from build123d import *

# Parameters (mm, degrees)
SKETCH1_W           = 5
SKETCH1_H           = 6.5
SKETCH1_W_2         = 29.5
SKETCH1_H_2         = 9.25
BOSS_EXTRUDE1_DEPTH = 1.62
FILLET1_R           = 10.16
SKETCH1_3_W         = 5
SKETCH1_3_H         = 6.5
BOSS_EXTRUDE2_DEPTH = 7
SKETCH2_R           = 1.5
CUT_EXTRUDE1_DEPTH  = 1.62
SKETCH3_W           = 20
SKETCH3_H           = 7
BOSS_EXTRUDE3_DEPTH = 6


with BuildPart() as part:
    # Sketch1 → Boss-Extrude1 (new body)
    # profile 1 of 7: a face of its own
    with BuildSketch(Plane(origin=(0, 0, 0), x_dir=(1, 0, 0), z_dir=(0, 1, 0))):
        Polygon((-38.5, 4.625), (-14.75, 4.625), (14.75, 4.625), (38.5, 4.625), (38.5, 13.875), (-38.5, 13.875), align=None)
        with Locations((-31.9999868, 9.25)):
            Rectangle(SKETCH1_W, SKETCH1_H, mode=Mode.SUBTRACT)
        with Locations((-15.9999934, 9.25)):
            Rectangle(SKETCH1_W, SKETCH1_H, mode=Mode.SUBTRACT)
        with Locations((0, 9.25)):
            Rectangle(SKETCH1_W, SKETCH1_H, mode=Mode.SUBTRACT)
        with Locations((15.9999934, 9.25)):
            Rectangle(SKETCH1_W, SKETCH1_H, mode=Mode.SUBTRACT)
        with Locations((31.9999868, 9.25)):
            Rectangle(SKETCH1_W, SKETCH1_H, mode=Mode.SUBTRACT)
    # profile 2 of 7: a face of its own
    with BuildSketch(Plane(origin=(0, 0, 0), x_dir=(1, 0, 0), z_dir=(0, 1, 0))):
        with Locations((-31.9999868, 9.25)):
            Rectangle(SKETCH1_W, SKETCH1_H)
    # profile 3 of 7: a face of its own
    with BuildSketch(Plane(origin=(0, 0, 0), x_dir=(1, 0, 0), z_dir=(0, 1, 0))):
        with Locations((-15.9999934, 9.25)):
            Rectangle(SKETCH1_W, SKETCH1_H)
    # profile 4 of 7: a face of its own
    with BuildSketch(Plane(origin=(0, 0, 0), x_dir=(1, 0, 0), z_dir=(0, 1, 0))):
        Rectangle(SKETCH1_W_2, SKETCH1_H_2)
    # profile 5 of 7: a face of its own
    with BuildSketch(Plane(origin=(0, 0, 0), x_dir=(1, 0, 0), z_dir=(0, 1, 0))):
        with Locations((0, 9.25)):
            Rectangle(SKETCH1_W, SKETCH1_H)
    # profile 6 of 7: a face of its own
    with BuildSketch(Plane(origin=(0, 0, 0), x_dir=(1, 0, 0), z_dir=(0, 1, 0))):
        with Locations((15.9999934, 9.25)):
            Rectangle(SKETCH1_W, SKETCH1_H)
    # profile 7 of 7: a face of its own
    with BuildSketch(Plane(origin=(0, 0, 0), x_dir=(1, 0, 0), z_dir=(0, 1, 0))):
        with Locations((31.9999868, 9.25)):
            Rectangle(SKETCH1_W, SKETCH1_H)
    extrude(amount=BOSS_EXTRUDE1_DEPTH)

    # Fillet1
    # the kernel refuses this fillet: 10.16 mm, written as the material it adds along each edge
    with BuildSketch(Plane(origin=(14.75, 0, -4.625), x_dir=(0, 0, 1), z_dir=(0, 1, 0))) as fillet1_piece_1:
        with BuildLine():
            CenterArc((10.16, 10.119164985), FILLET1_R, 180, 84.861306661)
            Line((0, 10.119164985), (-0.2032, 10.119164985))
            Line((-0.2032, 10.119164985), (-0.2032, 0))
            Line((-0.2032, 0), (0, -0.2032))
            ThreePointArc((0, -0.2032), (4.625, -0.2032), (9.2318, -0.2023833))
            Line((9.2318, -0.2023833), (9.25, 0))
        make_face()
    extrude(amount=1.62)
    with BuildSketch(Plane(origin=(-14.75, 0, -4.625), x_dir=(-1, 0, 0), z_dir=(0, 1, 0))) as fillet1_piece_2:
        with BuildLine():
            CenterArc((10.119164985, 10.16), FILLET1_R, 185.138693339, 84.861306661)
            Line((0, 9.25), (-0.2023833, 9.2318))
            ThreePointArc((-0.2023833, 9.2318), (-0.2032, 4.625), (-0.2032, 0))
            Line((-0.2032, 0), (0, -0.2032))
            Line((0, -0.2032), (10.119164985, -0.2032))
            Line((10.119164985, -0.2032), (10.119164985, 0))
        make_face()
    extrude(amount=1.62)

    # Sketch1<3> → Boss-Extrude2 (add)
    with BuildSketch(Plane(origin=(0, 0, 0), x_dir=(1, 0, 0), z_dir=(0, 1, 0))):
        with Locations((31.9999868, 9.25)):
            Rectangle(SKETCH1_3_W, SKETCH1_3_H)
        with Locations((15.9999934, 9.25)):
            Rectangle(SKETCH1_3_W, SKETCH1_3_H)
        with Locations((0, 9.25)):
            Rectangle(SKETCH1_3_W, SKETCH1_3_H)
        with Locations((-15.9999934, 9.25)):
            Rectangle(SKETCH1_3_W, SKETCH1_3_H)
        with Locations((-31.9999868, 9.25)):
            Rectangle(SKETCH1_3_W, SKETCH1_3_H)
    extrude(amount=-BOSS_EXTRUDE2_DEPTH)

    # Sketch2 → Cut-Extrude1 (cut)
    with BuildSketch(Plane(origin=(0, 1.62, 0), x_dir=(1, 0, 0), z_dir=(0, 1, 0))):
        with Locations(Location((-12.749999979, 1.624999898, 0), (0, 0, 270))):
            Circle(SKETCH2_R)
        with Locations(Location((12.749999979, 1.624999898, 0), (0, 0, 270))):
            Circle(SKETCH2_R)
    extrude(amount=-CUT_EXTRUDE1_DEPTH, mode=Mode.SUBTRACT)

    # Sketch3 → Boss-Extrude3 (add)
    with BuildSketch(Plane(origin=(0, 1.62, 0), x_dir=(1, 0, 0), z_dir=(0, 1, 0))):
        with Locations((0, -1.125)):
            Rectangle(SKETCH3_W, SKETCH3_H)
    extrude(amount=BOSS_EXTRUDE3_DEPTH)


solid = part.part
The model under review builds one solid part; all positions refer to its coordinate system, in mm. A direction names the side the tool comes from. Coordinates: 2 decimals unless noted, no trailing zeros. Write each loop counter-clockwise with the first axis right and the second up, starting at its lowest first coordinate (ties: lowest second). Pieces come first, ordered by that corner, then holes. Notation, with made-up numbers: (-10, 29) -> (13, 29) arc R25 cw to (13, 47) -> close; hole circle Ø2 at (76.5, -32). An arc over 180 degrees is marked (long way). Answer in a Markdown table with one row per item.
1. Wall thickness on probe 1 along X at (y, z) = (-4, -12.25); probe 2 along Z at (x, y) = (12.75, 0.6) (3 decimals); probe 3 along Y at (x, z) = (-15, -4.5): over which ranges is each line inside the solid? List them lowest first. Write a range as [from, to].
Answers below:
| item | result |
|---|---|
| probe 1 | x = [-34.5, -29.5], [-18.5, -13.5], [-2.5, 2.5], [13.5, 18.5], [29.5, 34.5] |
| probe 2 | z = [-13.875, -3.125], [-0.125, 4.625] |
| probe 3 | y = [0, 1.62] |
2. We need section D-D, the plane x = -4. State the section outline as (y, z) points (3 decimals), and give its area (3 significant figures).
Answers below:
| item | result |
|---|---|
| outline | (0, -13.875) -> (1.62, -13.875) -> (1.62, -2.375) -> (7.62, -2.375) -> (7.62, 4.625) -> (0, 4.625) -> close |
| area | 72.0 mm^2 |
3. Clearance check with flat-ended pins moving along their axes: pin 1 Ø6.5 at (y, z) = (5, -0.5) entering from -X; pin 2 Ø0.5 at (x, y) = (-33.5, 0.5) entering from +Z (3 decimals); pin 3 Ø1.5 at (x, y) = (-32.5, -3.5) entering from +Z. State where each tip first meets the part, or that it passes through.
Answers below:
| item | result |
|---|---|
| pin 1 | stops at x = -10 |
| pin 2 | stops at z = -4.625 |
| pin 3 | stops at z = -6 |
4. For faces 1 (the flat face through (2.5, -3, -9)), 2 (the flat face through (16, -3, -6)), 3 (the flat face through (32, 1, -4.625)), 4 (the flat face through (34.5, -3, -9)), 5 (the flat face through (-32, -3, -12.5)), list the 3-axis set-ups (+Z, -Z, +X, -X, +Y, -Y) from which the entire face can be reached by the end or side of a thin tool; tool diameter is ignored.
Answers below:
| item | result |
|---|---|
| face 1 | +Z, -Z, -Y |
| face 2 | +Z, +X, -X, -Y |
| face 3 | +Z, +X, +Y, -Y |
| face 4 | +Z, -Z, +X, -Y |
| face 5 | -Z, +X, -X, -Y |
5. We need section A-A, the plane y = -1. State the section outline as (x, z) points, and give its area (4 significant figures).
Answers below:
| item | result |
|---|---|
| outline | (-34.5, -12.5) -> (-29.5, -12.5) -> (-29.5, -6) -> (-34.5, -6) -> close; (-18.5, -12.5) -> (-13.5, -12.5) -> (-13.5, -6) -> (-18.5, -6) -> close; (-2.5, -12.5) -> (2.5, -12.5) -> (2.5, -6) -> (-2.5, -6) -> close; (13.5, -12.5) -> (18.5, -12.5) -> (18.5, -6) -> (13.5, -6) -> close; (29.5, -12.5) -> (34.5, -12.5) -> (34.5, -6) -> (29.5, -6) -> close |
| area | 162.5 mm^2 |
6. We need section C-C, the plane z = 0.75. State the section outline as (x, y) points.
Answers below:
| item | result |
|---|---|
| outline | (-15.91, 0) -> (15.91, 0) -> (15.91, 1.62) -> (10, 1.62) -> (10, 7.62) -> (-10, 7.62) -> (-10, 1.62) -> (-15.91, 1.62) -> close |
7. Draft analysis for pull direction X (two halves, no side actions). For faces 6 (the flat face through (29.5, -3, -9)), 7 (the flat face through (32, -3, -6)), 8 (the cylindrical face through (-17.937, 0.799, -1.893)), state which applies: +X half, -X half, draft (parallel to the pull), parting line (faces both ways), or undercut.
Answers below:
| item | result |
|---|---|
| face 6 | undercut |
| face 7 | draft |
| face 8 | -X half |
8. We need section B-B, the plane x = -12.75. State the section outline as (y, z) points (3 decimals), and give its area (3 significant figures).
Answers below:
| item | result |
|---|---|
| outline | (0, -13.875) -> (1.62, -13.875) -> (1.62, -3.125) -> (0, -3.125) -> close; (0, -0.125) -> (1.62, -0.125) -> (1.62, 4.625) -> (0, 4.625) -> close |
| area | 25.1 mm^2 |
